Work out the finished part from the listing and answer in its coordinate system (mm). A direction names the side the tool comes from. Round coordinates to 2 decimals unless told otherwise and drop trailing zeros. Write each loop counter-clockwise with the first axis right and the second up, starting at its lowest first coordinate (ties: lowest second). Pieces come first, ordered by that corner, then holes. Notation, with made-up numbers: M -23,81.5 L 22,81.5 A26 ccw 22,100.5 Z; hole C 21,-36 d5. An arc over 180 degrees is marked long. Answer in a Markdown table with one row per item.
```python
from build123d import *

# Parameters (mm, degrees)
ESBO_O1_R                = 1.6
ESBO_O1_R_2              = 3
RESSALTO_EXTRUS_O1_DEPTH = 6
FILETE1_R                = 5
FILETE2_R                = 2.6


with BuildPart() as part:
    # Esboço1 → Ressalto-extrusão1 (new body)
    with BuildSketch(Plane.XY):
        with BuildLine():
            Line((-7.5, 26.977225559), (-7.5, -38.489430519))
            Line((-7.5, -38.489430519), (7.5, -38.489430519))
            Line((7.5, -38.489430519), (7.5, 38.489430519))
            Line((7.5, 38.489430519), (-7.5, 38.489430519))
            Line((-7.5, 38.489430519), (-7.5, 33.031933101))
            ThreePointArc((-7.5, 33.031933101), (-4.54537196, 33.335220723), (-1.579224698, 33.489430519))
            ThreePointArc((-1.579224698, 33.489430519), (1.5, 30.570804942), (-1.418625577, 27.491580244))
            ThreePointArc((-1.418625577, 27.491580244), (-4.466722594, 27.322011321), (-7.5, 26.977225559))
        make_face()
        with Locations((0, -33.489430519)):
            Circle(ESBO_O1_R, mode=Mode.SUBTRACT)
        with Locations((0, -25.489430519)):
            Circle(ESBO_O1_R_2, mode=Mode.SUBTRACT)
        with Locations((0, -17.489430519)):
            Circle(ESBO_O1_R, mode=Mode.SUBTRACT)
    extrude(amount=RESSALTO_EXTRUS_O1_DEPTH)

    # Filete1
    filete1_edges = [part.edges().sort_by_distance(p)[0] for p in [
        (7.5, 38.489430519, 3),
        (7.5, -38.489430519, 3),
        (-7.5, -38.489430519, 3),
    ]]
    fillet(filete1_edges, radius=FILETE1_R)

    # Filete2
    filete2_edges = [part.edges().sort_by_distance(p)[0] for p in [
        (-7.5, 38.489430519, 3),
    ]]
    fillet(filete2_edges, radius=FILETE2_R)


solid = part.part
```
1. The part is cut by section A-A (x = 0.5). Determine the outline of the cut face in (y, z), plus the area to 3 significant figures.
Calculated:
| item | result |
|---|---|
| outline | M -38.49,0 L -35.01,0 L -35.01,6 L -38.49,6 Z; M -31.97,0 L -28.45,0 L -28.45,6 L -31.97,6 Z; M -22.53,0 L -19.01,0 L -19.01,6 L -22.53,6 Z; M -15.97,0 L 28.25,0 L 28.25,6 L -15.97,6 Z; M 32.73,0 L 38.49,0 L 38.49,6 L 32.73,6 Z |
| area | 363 mm² |
2. A tool of negligible diameter and unlimited length cuts with its end or side. For faces 4 (the flat face through (0, -38.489, 3)), 5 (the cylindrical face through (-4.59, 33.33, 2.96)), 6 (the cylindrical face through (-4.424, 27.326, 2.958)), from which of +Z, -Z, +X, -X, +Y, -Y can it reach the whole face along a straight path? Write none if from no direction.
Calculated:
| item | result |
|---|---|
| face 4 | +Z, -Z, +X, -X, -Y |
| face 5 | +Z, -Z |
| face 6 | +Z, -Z, -X |
3. The part is cut by section B-B (x = -6). Determine the outline of the cut face in (y, z).
Calculated:
| item | result |
|---|---|
| outline | M -37.06,0 L 27.17,0 L 27.17,6 L -37.06,6 Z; M 33.2,0 L 38.25,0 L 38.25,6 L 33.2,6 Z |
4. The part is cut by section C-C (z = 5.3). Determine the outline of the cut face in (x, y), plus the area to 3 significant figures.
Calculated:
| item | result |
|---|---|
| outline | M -7.5,-33.49 A5 ccw -2.5,-38.49 L 2.5,-38.49 A5 ccw 7.5,-33.49 L 7.5,33.49 A5 ccw 2.5,38.49 L -4.9,38.49 A2.6 ccw -7.5,35.89 L -7.5,33.03 A59 cw -1.58,33.49 A3 cw -1.42,27.49 A53 ccw -7.5,26.98 Z; hole C 0,-25.49 d6; hole C 0,-33.49 d3.2; hole C 0,-17.49 d3.2 |
| area | 1,040 mm² |
5. Consider line 1 along Y through (x, z) = (0, 3.25); line 2 along Y through (x, z) = (-2.75, 3.4); line 3 along Y through (x, z) = (-4, 2.7). Determine where each line is inside the solid, lowest interval first. Write a range as from..to.
Calculated:
| item | result |
|---|---|
| line 1 | y = -38.49..-35.09, -31.89..-28.49, -22.49..-19.09, -15.89..27.89, 33.09..38.49 |
| line 2 | y = -38.48..-26.69, -24.29..27.44, 33.45..38.49 |
| line 3 | y = -38.26..27.36, 33.37..38.49 |
6. Determine the mould class of faces 1 (the cylindrical face through (-0.65, -28.42, 2.96)), 2 (the flat face through (-1, 38.489, 3)), 3 (the cylindrical face through (-6.07, -36.99, 3.04)) for opening direction Y: released by +Y, released by -Y, zero draft, split by the parting line, or undercut.
Calculated:
| item | result |
|---|---|
| face 1 | undercut |
| face 2 | released by +Y |
| face 3 | released by -Y |
